The figure shows three views and two pictorial views of one solid part (mm, origin at its lowest corner). Answer the questions. A direction names the side the tool comes from. Round coordinates to 2 decimals unless told otherwise and drop trailing zeros. Order: outer loops, then holes, each group sorted by start corner. A loop starts at its lowest first (then second) coordinate and runs counter-clockwise, first axis right, second up. Notation, with made-up numbers: (-35, 33) - (17, 33) arc R11 ccw to (17, 52) - close; hole circle Ø11 at (-33.75, 80). An arc over 180 degrees is marked (long way). One line per question, with ' | ' between items. Start each with the question number.
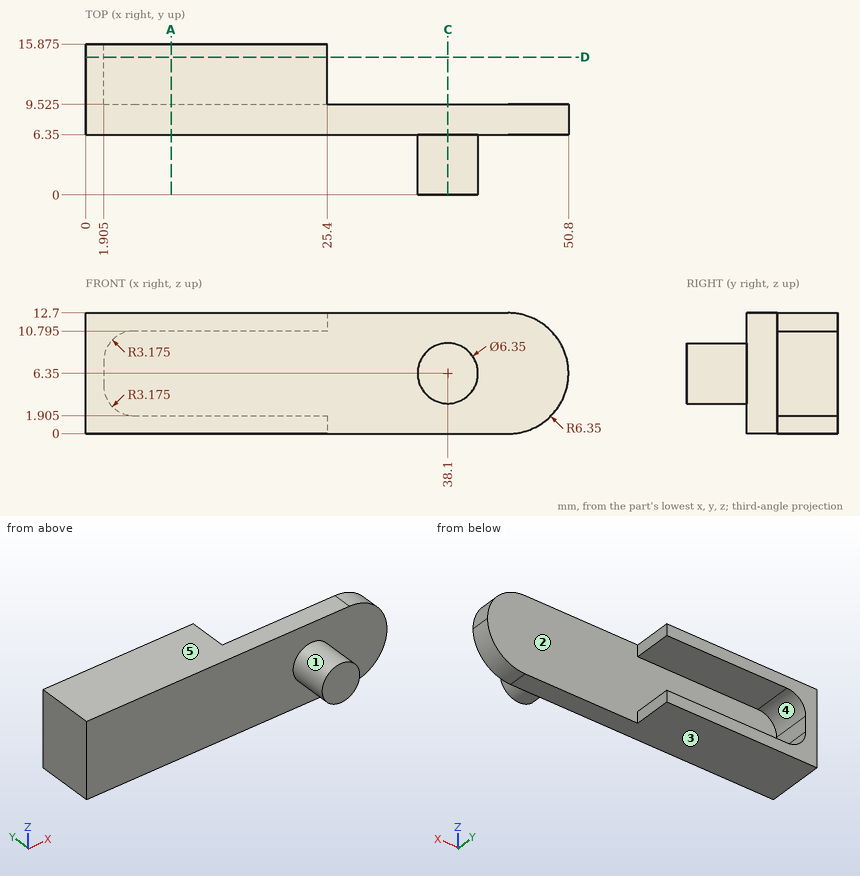
1) Determine the mould class of the marked faces 1, 2 and 3 for opening direction Z: released by +Z, released by -Z, zero draft, split by the parting line, or undercut.
2) Straight lines are drawn through the part: line 1 (Z direction, x = 25, y = 9.75) (3 decimals); line 2 (X direction, y = 10.75, z = 1.5); line 3 (Y direction, x = 9, z = 10.5) (3 decimals). For each, find the intervals that lie inside material, in ascending order.
3) Section C-C on x = 38.1 is taken. Give the vertices of the cut face in (y, z) (3 decimals).
4) Section D-D on y = 14.5 is taken. Give the vertices of the cut face in (x, z) (3 decimals).
5) For the marked faces 4 and 5, determine the directions among +Z, -Z, +X, -X, +Y, -Y from which every point of the face is accessible in a straight line to the end or side of a thin tool.
6) Flat-ended cylindrical pins translate along their axes: pin 1 (1 mm diameter, centred on y = 11.5, z = 11.5, fed in from +X); pin 2 (3 mm diameter, centred on y = 12, z = 7, fed in from +X). Find the tip coordinate at first contact, or state that the pin passes through.
7) Section A-A on x = 9 is taken. Give the vertices of the cut face in (y, z) (3 decimals).
Recorded:
1) face 1: split by the parting line | face 2: undercut | face 3: released by -Z
2) line 1: z = 0 to 1.905, 10.795 to 12.7 | line 2: x = 0 to 25.4 | line 3: y = 6.35 to 9.525
3) outline: (0, 3.175) - (6.35, 3.175) - (6.35, 0) - (9.525, 0) - (9.525, 12.7) - (6.35, 12.7) - (6.35, 9.525) - (0, 9.525) - close
4) outline: (0, 0) - (25.4, 0) - (25.4, 1.905) - (5.08, 1.905) arc R3.175 cw to (1.905, 5.08) - (1.905, 7.62) arc R3.175 cw to (5.08, 10.795) - (25.4, 10.795) - (25.4, 12.7) - (0, 12.7) - close
5) face 4: +X, +Y | face 5: +Z, +X, -X, +Y, -Y
6) pin 1: stops at x = 25.4 | pin 2: stops at x = 2.03
7) outline: (6.35, 0) - (15.875, 0) - (15.875, 1.905) - (9.525, 1.905) - (9.525, 10.795) - (15.875, 10.795) - (15.875, 12.7) - (6.35, 12.7) - close
